Here's how the part is built. I have some questions about the finished solid (model axes, mm). Give positions to 0.01 mm unless a question says otherwise; leave off trailing zeros. Write each loop counter-clockwise with the first axis right and the second up, starting at its lowest first coordinate (ties: lowest second). Pieces come first, ordered by that corner, then holes. Notation, with made-up numbers: (29.5, 52.25) -> (64.5, 52.25) arc R17 cw to (64.5, 83.25) -> close; hole circle Ø4 at (42.25, 80.25). An arc over 180 degrees is marked (long way). Use CSV: the item, a comma, the result in double quotes. Start each with the question number.
(1) Suppose I cut it at B-B on y = 0. List the corners of the cut face in (x, z) for me.
(2) I need wall thicknesses on L1, parallel to Z at x = -0.25, y = 1.5; L2, parallel to X at y = 1, z = 1; L3, parallel to X at y = -3.5, z = 6.25. Which ranges of each line are inside material? Lowest first, please. Write a range as [from, to].
(3) For pin 1 Ø1 at (x, z) = (-3, 3) entering from -Y; pin 2 Ø2 at (x, z) = (-2.5, 2) entering from +Y; pin 3 Ø5 at (x, z) = (3, 3.5) entering from -Y, each with a flat end and sliding along its axis, tell me the tip position at first contact or that it passes through.
(4) Suppose I cut it at C-C on z = 7. List the corners of the cut face in (x, y) for me, plus the area to 3 significant figures.
(5) Suppose I cut it at A-A on z = -4.5. List the corners of the cut face in (x, y) for me, plus the area to 3 significant figures.
Autodesk Inventor part; units mm, degrees
ref_plane "YZ Plane" through (0, 0, 0) normal (1, 0, 0) x (0, 1, 0)
ref_plane "XZ Plane" through (0, 0, 0) normal (0, 1, 0) x (-1, 0, 0)
ref_plane "XY Plane" through (0, 0, 0) normal (0, 0, 1) x (1, 0, 0)
sketch "Sketch1" plane through (0, 0, 0) normal (0, 0, 1) x (1, 0, 0)
  circle A0 centre (0, 0) radius 4.2426
extrude "Extrusion1" add sketch "Sketch1" along normal blind 10
fillet "Fillet1" radius 2 1 edges at (-4.2426, 0, 10)
sketch "Sketch2" plane through (0, 0, 0) normal (0, 0, -1) x (-1, 0, 0)
  line L0 (0, -4) -> (-0.2, -4)
  line L1 (-0.2, -4) -> (-0.2, -3.8)
  line L2 (-0.2, -3.8) -> (0, -3.8)
  line L3 (0, -3.8) -> (0, -4)
  line L4 (0, 4) -> (-0.2, 4)
  line L5 (-0.2, 4) -> (-0.2, 3.8)
  line L6 (-0.2, 3.8) -> (0, 3.8)
  line L7 (0, 3.8) -> (0, 4)
  point P0 (0, 0)
  dimension "d3" = 0.2
  dimension "d4" = 0.2
  dimension "d5" = 0.2
  dimension "d6" = 0.2
extrude "Extrusion2" add sketch "Sketch2" along normal blind 10 contours L0 L1 L2 L3
sketch "Sketch3" plane through (0, 0, 0) normal (0, 0, -1) x (-1, 0, 0)
  point P0 (0, 0)
sketch "Sketch4" plane through (0, 0, 0) normal (0, 0, -1) x (-1, 0, 0)
  line L0 (0, 4) -> (-0.2, 4)
  line L1 (-0.2, 4) -> (-0.2, 3.8)
  line L2 (-0.2, 3.8) -> (0, 3.8)
  line L3 (0, 3.8) -> (0, 4)
  point P0 (0, 0)
  dimension "d9" = 0.2
  dimension "d10" = 0.2
extrude "Extrusion3" add sketch "Sketch4" along normal blind 10
properties part number "bulb" material "Glass"
Geometry says:
1,outline,"(-4.24, 0) -> (4.24, 0) -> (4.24, 8) arc R2 ccw to (2.24, 10) -> (-2.24, 10) arc R2 ccw to (-4.24, 8) -> close"
2,L1,"[0, 10]"
2,L2,"[-4.12, 4.12]"
2,L3,"[-2.4, 2.4]"
3,pin 1,"y = -3.43"
3,pin 2,"y = 3.97"
3,pin 3,"y = -4.21"
4,outline,"circle Ø8.49 at (0, 0)"
4,area,"56.5 mm²"
5,outline,"(0, -4) -> (0.2, -4) -> (0.2, -3.8) -> (0, -3.8) -> close; (0, 3.8) -> (0.2, 3.8) -> (0.2, 4) -> (0, 4) -> close"
5,area,"0.0800 mm²"
